Part print with two shaded views. Sizes in mm from the minimum x, y, z corner. A direction names the side the tool comes from. Give positions to 0.01 mm unless a question says otherwise; leave off trailing zeros. Write each loop counter-clockwise with the first axis right and the second up, starting at its lowest first coordinate (ties: lowest second). Pieces come first, ordered by that corner, then holes.
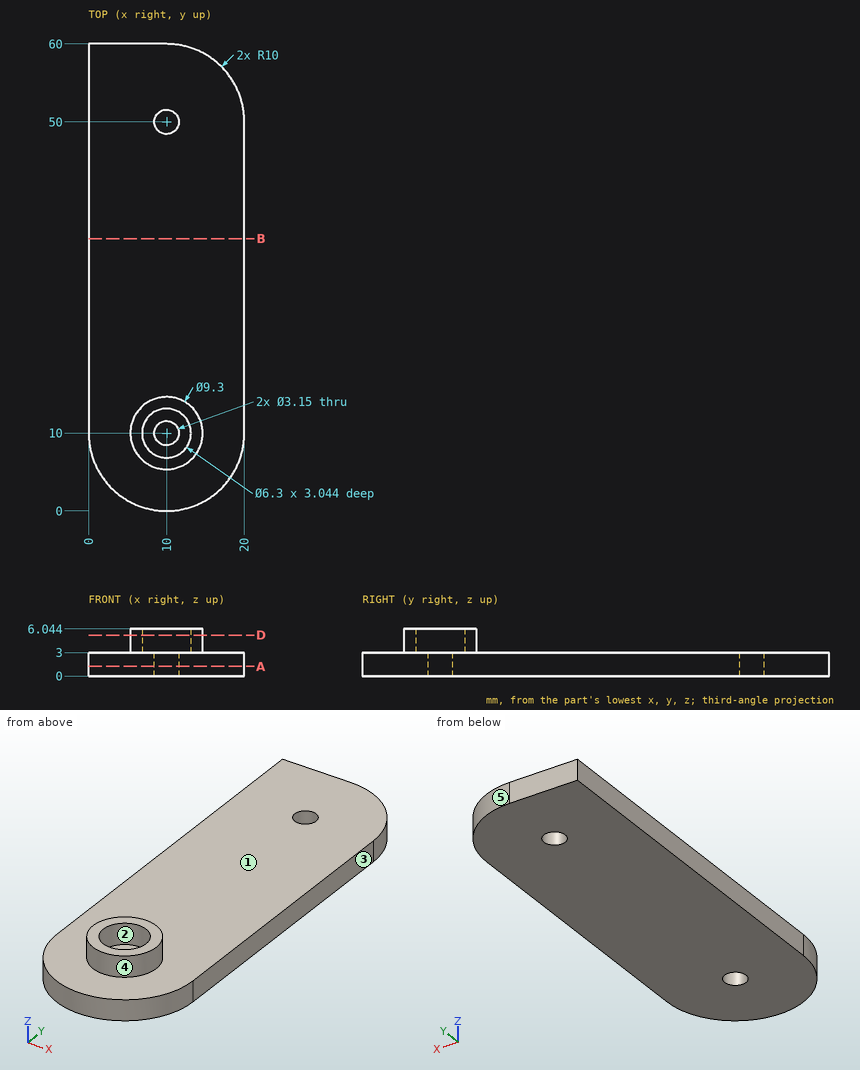
1) 3-axis set-ups, long thin cutter, end or side, ignore diameter. For the marked faces 4 and 5: which of +Z, -Z, +X, -X, +Y, -Y reach the whole face in a straight line?
Answers follow:
face 4: +Z
face 5: +Z, -Z, +X, +Y
2) Pin check, flat tips, straight feed: pin 1 Ø3 at (y, z) = (12.5, 5) entering from +X; pin 2 Ø1 at (x, y) = (3.5, 14) entering from +Z; pin 3 Ø3 at (x, z) = (11.5, 5) entering from +Y; pin 4 Ø1.5 at (x, y) = (14, 38.5) entering from -Z. Stop position of each tip, or through.
Answers follow:
pin 1: stops at x = 14.54
pin 2: stops at z = 3
pin 3: stops at y = 14.65
pin 4: stops at z = 0
3) Saw through at A-A, the plane z = 1.25. Count the separate pieces of the cut face and the enclosed holes in it, then the cut area to 3 significant figures.
Answers follow:
separate pieces: 1
enclosed holes: 2
area: 1,120 mm2
4) Wall check: L1, parallel to Y at x = 10, z = 2.4 (1 decimal); L2, parallel to Y at x = 9.75, z = 3.75; L3, parallel to Z at x = 4, y = 7. Give the ranges that are in metal, low to high.
Answers follow:
L1: y = 0 to 8.4, 11.6 to 48.4, 51.6 to 60
L2: y = 5.36 to 6.86, 13.14 to 14.64
L3: z = 0 to 3
5) Two-plate mould, pull along X, no slides. Class the marked faces 1, 2 and 3: +X half, -X half, draft (parallel to the pull), parting line (faces both ways), or undercut.
Answers follow:
face 1: draft
face 2: undercut
face 3: +X half
6) Saw through at D-D, the plane z = 5.25. Write the cut outline in (x, y).
Answers follow:
outline: circle Ø9.3 at (10, 10); hole circle Ø6.3 at (10, 10)
7) Saw through at B-B, the plane y = 35. Write the cut outline in (x, z).
Answers follow:
outline: (0, 0) - (20, 0) - (20, 3) - (0, 3) - close
